from build123d import *

# Parameters (mm, degrees)
SKETCH1_R           = 55
SKETCH1_R_2         = 42.5
BOSS_EXTRUDE1_DEPTH = 15
CUT_EXTRUDE1_DEPTH  = 80.214897589
CUT_EXTRUDE2_START  = -10
CUT_EXTRUDE2_DEPTH  = 10
SKETCH4_R           = 2.75
CUT_EXTRUDE3_DEPTH  = 84.858511792
FILLET2_R           = 2
CHAMFER1_SIZE       = 1.064458421
CHAMFER1_SIZE_2     = 1


with BuildPart() as part:
    # Sketch1 → Boss-Extrude1 (new body)
    with BuildSketch(Plane(origin=(0, 0, 0), x_dir=(1, 0, 0), z_dir=(0, 1, 0))):
        with Locations(Location((0, 0, 0), (0, 0, 270))):
            Circle(SKETCH1_R)
        with Locations(Location((0, 0, 0), (0, 0, 270))):
            Circle(SKETCH1_R_2, mode=Mode.SUBTRACT)
    extrude(amount=BOSS_EXTRUDE1_DEPTH)

    # Sketch2 → Cut-Extrude1 (cut, through all)
    with BuildSketch(Plane(origin=(0, 15, 0), x_dir=(1, 0, 0), z_dir=(0, 1, 0))):
        with BuildLine():
            Line((-2.5, 42.426406871), (-2.5, 54.94315244))
            ThreePointArc((-2.5, 54.94315244), (0, 55), (2.5, 54.94315244))
            Line((2.5, 54.94315244), (2.5, 42.426406871))
            ThreePointArc((2.5, 42.426406871), (0, 42.5), (-2.5, 42.426406871))
        make_face()
    extrude(amount=-CUT_EXTRUDE1_DEPTH, mode=Mode.SUBTRACT)

    # Sketch3 → Cut-Extrude2 (cut)
    with BuildSketch(Plane(origin=(0, 15, 0), x_dir=(1, 0, 0), z_dir=(0, 1, 0)).offset(CUT_EXTRUDE2_START)):
        with BuildLine():
            Line((-6.5, 54.614558499), (-6.5, 44.614558499))
            Line((-6.5, 44.614558499), (-32.164284074, 44.614558499))
            ThreePointArc((-32.164284074, 44.614558499), (-19.96826772, 51.247129522), (-6.5, 54.614558499))
        make_face()
        with BuildLine():
            Line((6.5, 44.614558499), (32.164284074, 44.614558499))
            ThreePointArc((32.164284074, 44.614558499), (19.96826772, 51.247129522), (6.5, 54.614558499))
            Line((6.5, 54.614558499), (6.5, 44.614558499))
        make_face()
    extrude(amount=CUT_EXTRUDE2_DEPTH, mode=Mode.SUBTRACT)

    # Sketch4 → Cut-Extrude3 (cut, through all)
    with BuildSketch(Plane.ZY.offset(6.5)):
        with Locations((-49.614558499, 10)):
            Circle(SKETCH4_R)
    extrude(amount=-CUT_EXTRUDE3_DEPTH, mode=Mode.SUBTRACT)

    # Fillet2
    fillet2_edges = [part.edges().sort_by_distance(p)[0] for p in [
        (-19.332142037, 5, -44.614558499),
        (19.332142037, 5, -44.614558499),
    ]]
    fillet(fillet2_edges, radius=FILLET2_R)

    # Chamfer1
    # the kernel refuses this chamfer: 1.064458421, 1 mm, written as the material it takes off along each edge
    with BuildSketch(Plane(origin=(2.5, 17.741623876, -42.426406871), x_dir=(0, 0, -1), z_dir=(0, -1, 0))) as chamfer1_piece_1:
        with BuildLine():
            Line((CHAMFER1_SIZE, 0), (-0.071563276, 1.009590298))
            ThreePointArc((-0.071563276, 1.009590298), (-0.033856315, 0.520208167), (0, 0))
            Line((0, 0), (CHAMFER1_SIZE, 0))
        make_face()
    extrude(amount=20.483247753, mode=Mode.SUBTRACT)
    with BuildSketch(Plane(origin=(-2.5, 17.781296166, -42.426406871), x_dir=(0, 0, -1), z_dir=(0, -1, 0))) as chamfer1_piece_2:
        with BuildLine():
            Line((CHAMFER1_SIZE_2, 0), (-0.077221697, -1.077221697))
            ThreePointArc((-0.077221697, -1.077221697), (-0.03634309, -0.554912866), (0, 0))
            Line((0, 0), (CHAMFER1_SIZE_2, 0))
        make_face()
    extrude(amount=20.562592333, mode=Mode.SUBTRACT)
    # the kernel refuses this chamfer: 1.064458421, 1 mm, written as the material it takes off along each edge
    with BuildSketch(Plane(origin=(0, 0, 0), x_dir=(-0.023665071979994685, 0, -0.9997199429681204), z_dir=(0.9997199429681204, 0, -0.023665071979994685))) as chamfer1_2_piece_1:
        Polygon((42.5 + CHAMFER1_SIZE_2, 0), (42.5, CHAMFER1_SIZE_2), (42.5, 0), align=None)
    revolve(axis=Axis((0, 0, 0), (0, 1, 0)), revolution_arc=178.643964662, mode=Mode.SUBTRACT)
    with BuildSketch(Plane(origin=(0, 15, 0), x_dir=(0, 0, 1), z_dir=(-1, 0, 0))) as chamfer1_2_piece_2:
        Polygon((42.5 + CHAMFER1_SIZE_2, 0), (42.5, -CHAMFER1_SIZE_2), (42.5, 0), align=None)
    revolve(axis=Axis((0, 15, 0), (0, 1, 0)), revolution_arc=178.735465076, mode=Mode.SUBTRACT)
    with BuildSketch(Plane(origin=(0, 15, 0), x_dir=(-0.023665071979993797, 0, -0.9997199429681204), z_dir=(0.9997199429681204, 0, -0.023665071979993797))) as chamfer1_2_piece_3:
        Polygon((42.5 + CHAMFER1_SIZE_2, 0), (42.5, -CHAMFER1_SIZE_2), (42.5, 0), align=None)
    revolve(axis=Axis((0, 15, 0), (0, 1, 0)), revolution_arc=178.643964662, mode=Mode.SUBTRACT)
    with BuildSketch(Plane(origin=(0, 0, 0), x_dir=(0, 0, 1), z_dir=(-1, 0, 0))) as chamfer1_2_piece_4:
        Polygon((42.5 + CHAMFER1_SIZE_2, 0), (42.5, CHAMFER1_SIZE_2), (42.5, 0), align=None)
    revolve(axis=Axis((0, 0, 0), (0, 1, 0)), revolution_arc=178.735465076, mode=Mode.SUBTRACT)


solid = part.part
Geometry: final body of the model. Coordinates: model frame, mm. A direction names the side the tool comes from. Coordinates: 2 decimals unless noted, no trailing zeros. Write each loop counter-clockwise with the first axis right and the second up, starting at its lowest first coordinate (ties: lowest second). Pieces come first, ordered by that corner, then holes. Notation, with made-up numbers: (23, 76) - (59, 76) arc R31 ccw to (59, 103) - close; hole circle Ø9 at (-32.5, 88.25). An arc over 180 degrees is marked (long way). Return JSON: item names as keys, results as strings.
Item 1: Section query B-B (y = 10). Output: boundary loops of the cut face in (x, z), and give its area (3 significant figures).
Completed:
{"outline": "(-32.16, -44.61) - (-6.5, -44.61) - (-6.5, -46.86) - (-2.5, -46.86) - (-2.5, -43.43) - (-3.58, -42.35) arc R42.5 cw (long way) to (3.51, -42.35) - (2.5, -43.49) - (2.5, -46.86) - (6.5, -46.86) - (6.5, -44.61) - (32.16, -44.61) arc R55 ccw (long way) to start; (-6.5, -54.61) arc R55 ccw to (-2.5, -54.94) - (-2.5, -52.36) - (-6.5, -52.36) - close; (2.5, -54.94) arc R55 ccw to (6.5, -54.61) - (6.5, -52.36) - (2.5, -52.36) - close", "area": "3,400 mm2"}
Item 2: Line query: L1, parallel to X at y = 4.25, z = 0; L2, parallel to Z at x = 0, y = 9; L3, parallel to Z at x = 31, y = 5. Output: solid intervals per line, ascending.
Completed:
{"L1": "x = -55 to -42.5, 42.5 to 55", "L2": "z = 42.5 to 55", "L3": "z = -45.43 to -29.07, 29.07 to 45.43"}
Item 3: Pull-direction query (Z, two-part tool) for faces 5 (the face through (-2.38, 7.4, 54.95)), 6 (the face through (-4.5, 11.9, -51.6)), 7 (the face through (-19, 11, -44.615)), 8 (the face through (6.5, 12, -52)); classes: +Z half, -Z half, draft (parallel to the pull), parting line (faces both ways), or undercut.
Completed:
{"face 5": "parting line", "face 6": "undercut", "face 7": "-Z half", "face 8": "draft"}
Item 4: Reachability of faces 1 (the face through (-15, 5, -50)), 2 (the face through (2.5, 6, -49)), 3 (the face through (-1.785, 7.409, 42.462)), 4 (the face through (15, 5, -50)) from +Z, -Z, +X, -X, +Y, -Y: full face, straight path, thin tool, end or side. Return the list, or none.
Completed:
{"face 1": "-Z, -X, +Y", "face 2": "-Z, +Y, -Y", "face 3": "+Y, -Y", "face 4": "-Z, +X, +Y"}
Item 5: Section query A-A (z = 0). Output: boundary loops of the cut face in (x, y).
Completed:
{"outline": "(-55, 0) - (-43.5, 0) - (-42.5, 1) - (-42.5, 14) - (-43.5, 15) - (-55, 15) - close; (42.5, 1) - (43.5, 0) - (55, 0) - (55, 15) - (43.5, 15) - (42.5, 14) - close"}
Item 6: Pin query (flat end, axial travel): pin 1 Ø2.5 at (x, z) = (18.5, -51.5) entering from +Y; pin 2 Ø4 at (x, y) = (25, 6) entering from -Z; pin 3 Ø3.5 at (y, z) = (4.5, -51.5) entering from -X. Return the tip coordinate at first contact, or that it passes through.
Completed:
{"pin 1": "stops at y = 5", "pin 2": "stops at z = -49.84", "pin 3": "stops at x = -23.45"}
